Model file for the job. Use its own axes, mm. Face numbers are marked on the shaded views. A direction names the side the tool comes from. Coordinates: 2 decimals unless noted, no trailing zeros. Order: outer loops, then holes, each group sorted by start corner. A loop starts at its lowest first (then second) coordinate and runs counter-clockwise, first axis right, second up.
from build123d import *

# Parameters (mm, degrees)
SKETCH1_W                = 22.5
SKETCH1_H                = 11.8
BOSS_EXTRUDE1_DEPTH      = 22.7
BOSS_EXTRUDE2_DEPTH      = 4.7
BOSS_EXTRUDE2_DEPTH_BACK = 27.4
SKETCH2_W                = 11.8
SKETCH2_H                = 2.5
BOSS_EXTRUDE3_DEPTH      = 4
SKETCH4_R                = 2.3
BOSS_EXTRUDE4_DEPTH      = 3.2


with BuildPart() as part:
    # Sketch1 → Boss-Extrude1 (new body)
    with BuildSketch(Plane(origin=(0, 0, 0), x_dir=(1, 0, 0), z_dir=(0, 1, 0))):
        Rectangle(SKETCH1_W, SKETCH1_H)
    extrude(amount=BOSS_EXTRUDE1_DEPTH)

    # Sketch2 → Boss-Extrude2 (add, two sides: drawn at the far end of the back side and taken through both)
    with BuildSketch(Plane.ZY.offset(11.25).offset(-BOSS_EXTRUDE2_DEPTH_BACK)):
        with Locations((0, 17.15)):
            Rectangle(SKETCH2_W, SKETCH2_H)
    extrude(amount=BOSS_EXTRUDE2_DEPTH + BOSS_EXTRUDE2_DEPTH_BACK)

    # Sketch3 → Boss-Extrude3 (add)
    with BuildSketch(Plane(origin=(0, 22.7, 0), x_dir=(1, 0, 0), z_dir=(0, 1, 0))):
        with BuildLine():
            ThreePointArc((0.137725696, 2.443247676), (-11.132613287, 0), (0.137725696, -2.443247676))
            ThreePointArc((0.137725696, -2.443247676), (3.167386713, 0), (0.137725696, 2.443247676))
        make_face()
    extrude(amount=BOSS_EXTRUDE3_DEPTH)

    # Sketch4 → Boss-Extrude4 (add)
    with BuildSketch(Plane(origin=(0, 26.7, 0), x_dir=(1, 0, 0), z_dir=(0, 1, 0))):
        with Locations(Location((-5.232613287, 0, 0), (0, 0, 270))):
            Circle(SKETCH4_R)
    extrude(amount=BOSS_EXTRUDE4_DEPTH)


solid = part.part
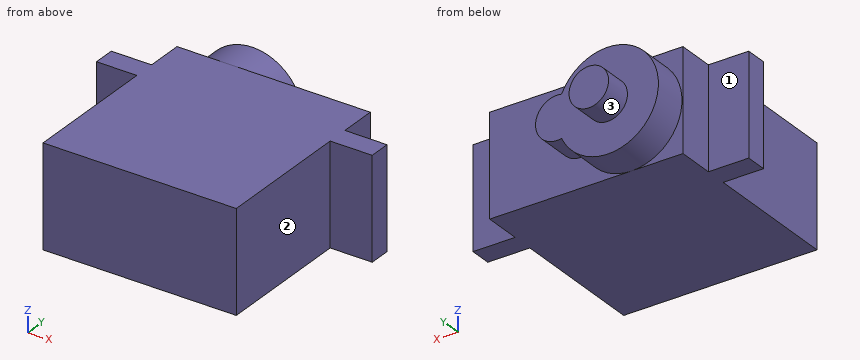
Q1. Which spindle directions (+Z, -Z, +X, -X, +Y, -Y) get a long thin tool onto all of the face, cutting with end or side? Do the marked faces 1, 2 and 3. Say none if no direction does.
Established:
face 1: +Z, -Z, -X, +Y
face 2: +Z, -Z, +X, -Y
face 3: +Y
Q2. Probe line 1 (Y direction, x = -13, z = 4); line 2 (X direction, y = 10, z = -4.75); line 3 (Z direction, x = 0.5, y = 25). List the from-to ranges inside material, lowest first.
Established:
line 1: y = 15.9 to 18.4
line 2: x = -11.25 to 11.25
line 3: z = -2.49 to 2.49
Q3. Cut at A-A, the plane z = 0. List the corners of the cut face in (x, y).
Established:
outline: (-15.95, 15.9) - (-11.25, 15.9) - (-11.25, 0) - (11.25, 0) - (11.25, 15.9) - (16.15, 15.9) - (16.15, 18.4) - (11.25, 18.4) - (11.25, 22.7) - (3.17, 22.7) - (3.17, 26.7) - (-2.93, 26.7) - (-2.93, 29.9) - (-7.53, 29.9) - (-7.53, 26.7) - (-11.13, 26.7) - (-11.13, 22.7) - (-11.25, 22.7) - (-11.25, 18.4) - (-15.95, 18.4) - close
Q4. Cut at B-B, the plane y = 27.5. List the corners of the cut face in (x, z), plus the area to 3 significant figures.
Established:
outline: circle Ø4.6 at (-5.23, 0)
area: 16.6 mm2
Q5. Drop flat-ended pins along their axis: P1, Ø1, axis at y = 26, z = -2, coming from the +X side; P2, Ø4, axis at x = -13, z = 3, coming from the -Y side; P3, Ø1.3, axis at y = 19.5, z = -2, coming from the -X side; P4, Ø5.5, axis at x = 15, z = 2.5, coming from the -Y side. Give the stop position or say it passes through.
Established:
P1: stops at x = 2.67
P2: stops at y = 0
P3: stops at x = -11.25
P4: stops at y = 15.9
Q6. Cut at D-D, the plane y = 10.5. List the corners of the cut face in (x, z), plus the area to 4 significant figures.
Established:
outline: (-11.25, -5.9) - (11.25, -5.9) - (11.25, 5.9) - (-11.25, 5.9) - close
area: 265.5 mm2
Q7. Cut at C-C, the plane x = -0.5. List the corners of the cut face in (y, z), plus the area to 3 significant figures.
Established:
outline: (0, -5.9) - (22.7, -5.9) - (22.7, -3.52) - (26.7, -3.52) - (26.7, 3.52) - (22.7, 3.52) - (22.7, 5.9) - (0, 5.9) - close
area: 296 mm2
